Can you work these out from the model? Positions are in its coordinate system, mm. Face numbers are marked on the shaded views. A direction names the side the tool comes from. Give positions to 0.01 mm unless a question says otherwise; leave off trailing zeros. Order: outer loops, then holes, each group sorted by start corner. A loop starts at its lowest first (then second) coordinate and runs counter-clockwise, first axis right, second up. Notation, with made-up numbers: (36.25, 53) - (40.25, 53) arc R14 ccw to (40.25, 57) - close; hole circle Ø4 at (38, -25). An arc over 180 degrees is marked (long way). Return JSON: item names as keys, results as strings.
```python
from build123d import *

# Parameters (mm, degrees)
SKETCH1_W           = 232.4
SKETCH1_H           = 85
BOSS_EXTRUDE1_DEPTH = 150
CUT_EXTRUDE1_DEPTH  = 150
CUT_EXTRUDE2_DEPTH  = 150
SKETCH4_R           = 11.5
SKETCH4_R_2         = 2.2
SKETCH4_R_3         = 4.5
CUT_EXTRUDE3_DEPTH  = 280.849977667
SKETCH5_R           = 10
SKETCH5_R_2         = 2.2
CUT_EXTRUDE4_DEPTH  = 189.341949655
SKETCH6_R           = 2.2
CUT_EXTRUDE5_DEPTH  = 221.699143461


with BuildPart() as part:
    # Sketch1 → Boss-Extrude1 (new body)
    with BuildSketch(Plane(origin=(0, 0, 0), x_dir=(1, 0, 0), z_dir=(0, 1, 0))):
        Rectangle(SKETCH1_W, SKETCH1_H)
    extrude(amount=BOSS_EXTRUDE1_DEPTH)

    # Sketch2 → Cut-Extrude1 (cut)
    with BuildSketch(Plane.XY.offset(42.5)):
        Polygon((-116.2, 0), (-116.2, 60), (-42.5, 0), align=None)
        Polygon((116.2, 60), (42.5, 0), (116.2, 0), align=None)
    extrude(amount=-CUT_EXTRUDE1_DEPTH, mode=Mode.SUBTRACT)

    # Sketch3 → Cut-Extrude2 (cut)
    with BuildSketch(Plane.XY.offset(42.5)):
        Polygon((-108.2, 142), (-108.2, 150), (108.2, 150), (108.2, 142), (108.2, 63.803007219), (39.655306133, 8), (-39.655306133, 8), (-108.2, 63.803007219), align=None)
    extrude(amount=-CUT_EXTRUDE2_DEPTH, mode=Mode.SUBTRACT)

    # Sketch4 → Cut-Extrude3 (cut, through all)
    with BuildSketch(Plane.ZY.offset(116.2)):
        with Locations((0, 110)):
            Circle(SKETCH4_R)
        with Locations((0, 139)):
            Circle(SKETCH4_R_2)
        with Locations((0, 129.25)):
            Circle(SKETCH4_R_3)
        with Locations((29.444863729, 88)):
            Circle(SKETCH4_R_2)
        with Locations((-29.444863729, 88)):
            Circle(SKETCH4_R_2)
    extrude(amount=-CUT_EXTRUDE3_DEPTH, mode=Mode.SUBTRACT)

    # Sketch5 → Cut-Extrude4 (cut, through all)
    with BuildSketch(Plane(origin=(0, 8, 0), x_dir=(1, 0, 0), z_dir=(0, 1, 0))):
        with Locations(Location((0, 0, 0), (0, 0, 270))):
            Circle(SKETCH5_R)
        with Locations(Location((0, 22.5, 0), (0, 0, 270))):
            Circle(SKETCH5_R_2)
        with Locations(Location((15.909902577, 15.909902577, 0), (0, 0, 270))):
            Circle(SKETCH5_R_2)
        with Locations(Location((22.5, 0, 0), (0, 0, 270))):
            Circle(SKETCH5_R_2)
        with Locations(Location((15.909902577, -15.909902577, 0), (0, 0, 270))):
            Circle(SKETCH5_R_2)
        with Locations(Location((0, -22.5, 0), (0, 0, 270))):
            Circle(SKETCH5_R_2)
        with Locations(Location((-15.909902577, -15.909902577, 0), (0, 0, 270))):
            Circle(SKETCH5_R_2)
        with Locations(Location((-22.5, 0, 0), (0, 0, 270))):
            Circle(SKETCH5_R_2)
        with Locations(Location((-15.909902577, 15.909902577, 0), (0, 0, 270))):
            Circle(SKETCH5_R_2)
    extrude(amount=-CUT_EXTRUDE4_DEPTH, mode=Mode.SUBTRACT)

    # Sketch6 → Cut-Extrude5 (cut, through all)
    with BuildSketch(Plane(origin=(-16.940351141, -20.808397985, 0), x_dir=(0.7755020970674419, -0.631344990828311, 0), z_dir=(-0.631344990828311, -0.7755020970674419, 0))):
        with Locations((-102.994043129, 32.5)):
            Circle(SKETCH6_R)
        with Locations((-87.994043129, 32.5)):
            Circle(SKETCH6_R)
        with Locations((-72.994043129, 32.5)):
            Circle(SKETCH6_R)
        with Locations((-57.994043129, 32.5)):
            Circle(SKETCH6_R)
        with Locations((-57.994043129, -32.5)):
            Circle(SKETCH6_R)
        with Locations((-72.994043129, -32.5)):
            Circle(SKETCH6_R)
        with Locations((-87.994043129, -32.5)):
            Circle(SKETCH6_R)
        with Locations((-102.994043129, -32.5)):
            Circle(SKETCH6_R)
    cut_extrude5 = extrude(amount=-CUT_EXTRUDE5_DEPTH, mode=Mode.SUBTRACT)

    # Mirror1: Cut-Extrude5 across plane
    add(cut_extrude5.mirror(Plane(origin=(0, 0, 0), x_dir=(0, 0, 1), z_dir=(1, 0, 0))), mode=Mode.SUBTRACT)


solid = part.part
```
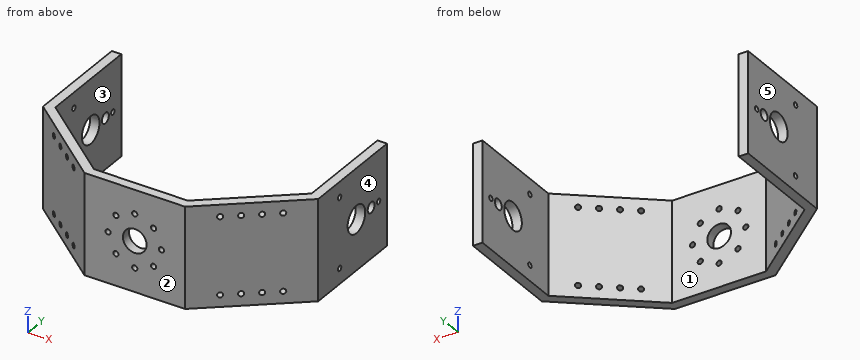
1. Suppose I cut it at C-C (y = 57). List the corners of the cut face in (x, z) for me (3 decimals).
Checks:
{"outline": "(-112.515, -42.5) - (-99.844, -42.5) - (-99.844, 42.5) - (-112.515, 42.5) - close; (99.844, -42.5) - (112.515, -42.5) - (112.515, 42.5) - (99.844, 42.5) - close"}
2. If I drill on L1, parallel to X at y = 84.5, z = 9; L2, parallel to X at y = 5, z = 0; L3, parallel to X at y = 46, z = -31, over which ranges is the centre line in solid material (lowest first)? Write a range as [from, to].
Checks:
{"L1": "[-116.2, -108.2], [108.2, 116.2]", "L2": "[-48.64, -24.7], [-20.3, -10], [10, 20.3], [24.7, 48.64]", "L3": "[-99, -97.44], [-93.29, -86.33], [86.33, 93.29], [97.44, 99]"}
3. On a 3-axis mill with a long thin cutter (end or side, diameter ignored), from which of +Z, -Z, +X, -X, +Y, -Y can I reach the whole of each face in a straight line? I mean the marked faces 1 and 2. Say none if no direction works.
Checks:
{"face 1": "+Z, -Z, +Y", "face 2": "+Z, -Z, +X, -X, -Y"}
4. For pin 1 Ø10 at (x, y) = (11, 16.5) entering from +Z; pin 2 Ø5.5 at (x, z) = (-15.91, 15.91) entering from +Y; pin 3 Ø5 at (y, z) = (88, -29.44) entering from -X, each with a flat end and sliding along its axis, tell me the tip position at first contact or that it passes through.
Checks:
{"pin 1": "through", "pin 2": "y = 8", "pin 3": "x = -116.2"}
5. Suppose I cut it at B-B (y = 82). List the corners of the cut face in (x, z) for me, plus the area to 3 significant figures.
Checks:
{"outline": "(-116.2, -42.5) - (-108.2, -42.5) - (-108.2, 42.5) - (-116.2, 42.5) - close; (108.2, -42.5) - (116.2, -42.5) - (116.2, 42.5) - (108.2, 42.5) - close", "area": "1,360 mm^2"}
6. Suppose I cut it at A-A (y = 110). List the corners of the cut face in (x, z) for me, plus the area to 3 significant figures.
Checks:
{"outline": "(-116.2, -42.5) - (-108.2, -42.5) - (-108.2, -11.5) - (-116.2, -11.5) - close; (-116.2, 11.5) - (-108.2, 11.5) - (-108.2, 42.5) - (-116.2, 42.5) - close; (108.2, -42.5) - (116.2, -42.5) - (116.2, -11.5) - (108.2, -11.5) - close; (108.2, 11.5) - (116.2, 11.5) - (116.2, 42.5) - (108.2, 42.5) - close", "area": "992 mm^2"}
7. Thinking about a two-plate mould opening in X: for the marked faces 3, 4 and 5, which applies, +X half, -X half, draft (parallel to the pull), parting line (faces both ways), or undercut?
Checks:
{"face 3": "undercut", "face 4": "+X half", "face 5": "-X half"}
